Here's how the part is built. I have some questions about the finished solid (model axes, mm). Face numbers are marked on the shaded views. A direction names the side the tool comes from. Round coordinates to 2 decimals unless told otherwise and drop trailing zeros. Loops run counter-clockwise (first coordinate to the right, second up) from the corner with the lowest first, then second, coordinate; pieces in that order, holes last. Notation, with made-up numbers: M 35.5,46 L 84.5,46 A13 ccw 84.5,60 Z; hole C -16,-13 d1. An arc over 180 degrees is marked long. Answer as a JSON object with one key per item and string values.
from build123d import *

# Parameters (mm, degrees)
SKETCH_1_R      = 7
SKETCH_1_R_2    = 2.5
EXTRUDE_1_DEPTH = 2


with BuildPart() as part:
    # 草图1 → 凸台-拉伸1 (new, symmetric)
    with BuildSketch(Plane.XY):
        Circle(SKETCH_1_R)
        Circle(SKETCH_1_R_2, mode=Mode.SUBTRACT)
    extrude(amount=EXTRUDE_1_DEPTH, both=True)

    # 草图2 → 旋转1 (revolve)
    with BuildSketch(Plane(origin=(0, 0, 0), x_dir=(0, 0, -1), z_dir=(1, 0, 0))):
        with BuildLine():
            ThreePointArc((-3, 3.5), (0, 4.609772229), (3, 3.5))
            Line((3, 3.5), (3, 2.5))
            Line((3, 2.5), (-3, 2.5))
            Line((-3, 2.5), (-3, 3.5))
        make_face()
    revolve(axis=Axis((0, 0, 0), (0, 0, 1)))


solid = part.part
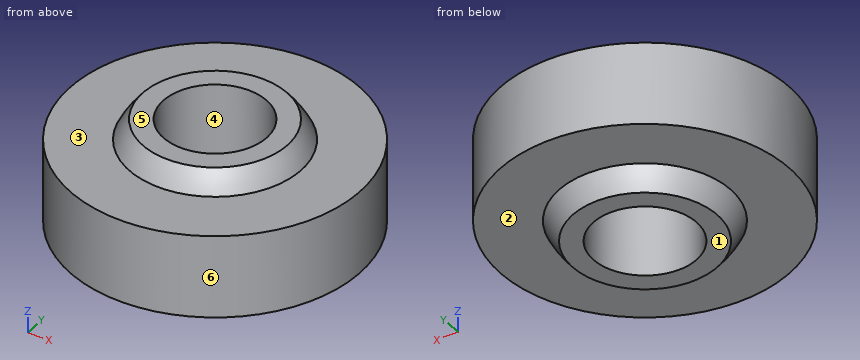
Item 1: I want a section at D-D on y = 2.75. List the corners of the cut face in (x, z) for me, plus the area to 3 significant figures.
Solution:
{"outline": "M -6.44,-2 L -3.11,-2 A3.7 ccw -2.17,-3 L 2.17,-3 A3.7 ccw 3.11,-2 L 6.44,-2 L 6.44,2 L 3.11,2 A3.7 ccw 2.17,3 L -2.17,3 A3.7 ccw -3.11,2 L -6.44,2 Z", "area": "62.3 mm2"}
Item 2: I want a section at C-C on z = -0.1. List the corners of the cut face in (x, y) for me, plus the area to 3 significant figures.
Solution:
{"outline": "C 0,0 d14; hole C 0,0 d5", "area": "134 mm2"}
Item 3: For the marked faces 1, 2 and 3, which set-ups out of +Z, -Z, +X, -X, +Y, -Y let a thin tool reach every point of the face, with its end or its side?
Solution:
{"face 1": "-Z, +X, -X, +Y, -Y", "face 2": "-Z", "face 3": "+Z"}
Item 4: I want a section at A-A on x = 0. List the corners of the cut face in (y, z) for me.
Solution:
{"outline": "M -7,-2 L -4.15,-2 A4.61 ccw -3.5,-3 L -2.5,-3 L -2.5,3 L -3.5,3 A4.61 ccw -4.15,2 L -7,2 Z; M 2.5,-3 L 3.5,-3 A4.61 ccw 4.15,-2 L 7,-2 L 7,2 L 4.15,2 A4.61 ccw 3.5,3 L 2.5,3 Z"}
Item 5: If I drill on L1, parallel to Y at x = 0, z = 0.2; L2, parallel to Z at x = 5.75, y = -2.25; L3, parallel to X at y = -1.5, z = -1.75, over which ranges is the centre line in solid material (lowest first)? Write a range as from..to.
Solution:
{"L1": "y = -7..-2.5, 2.5..7", "L2": "z = -2..2", "L3": "x = -6.84..-2, 2..6.84"}
Item 6: I want a section at B-B on y = 0.25. List the corners of the cut face in (x, z) for me.
Solution:
{"outline": "M -7,-2 L -4.15,-2 A4.6 ccw -3.49,-3 L -2.49,-3 L -2.49,3 L -3.49,3 A4.6 ccw -4.15,2 L -7,2 Z; M 2.49,-3 L 3.49,-3 A4.6 ccw 4.15,-2 L 7,-2 L 7,2 L 4.15,2 A4.6 ccw 3.49,3 L 2.49,3 Z"}
Item 7: For P1, Ø5, axis at x = -1, y = 4, coming from the -Z side; P2, Ø2, axis at x = 4.5, z = -2, coming from the +Y side, each with a flat end and sliding along its axis, tell me the tip position at first contact or that it passes through.
Solution:
{"P1": "stops at z = -3", "P2": "stops at y = 6.06"}
Item 8: We'd pull the mould along Y, two halves only. Please class the marked faces 4, 5 and 6: +Y half, -Y half, draft (parallel to the pull), parting line (faces both ways), or undercut.
Solution:
{"face 4": "undercut", "face 5": "draft", "face 6": "parting line"}
